For this review, use the dimensioned drawing (mm, ordinates from the lowest corner) and the shaded views. A direction names the side the tool comes from. Coordinates: 2 decimals unless noted, no trailing zeros. Loops run counter-clockwise (first coordinate to the right, second up) from the corner with the lowest first, then second, coordinate; pieces in that order, holes last. Notation, with made-up numbers: (16, 6.5) - (33, 6.5) arc R17 ccw to (33, 33.5) - close; hole circle Ø3 at (-22, 50.25). An arc over 180 degrees is marked (long way). Answer in a Markdown table with one row per item. Add a question column.
(1) We need section C-C, the plane x = 9. Write out the cut boundary in (y, z).
(2) We need section B-B, the plane x = 12.7. Write out the cut boundary in (y, z).
(3) We need section A-A, the plane y = 1.25. Write out the cut boundary in (x, z).
(4) For the marked faces 4 and 5, list the 3-axis set-ups (+Z, -Z, +X, -X, +Y, -Y) from which the entire face can be reached by the end or side of a thin tool; tool diameter is ignored.
(5) The part is to be moulded in two halves that separate along X. For the marked faces 1, 2 and 3, say which applies: released by +X, released by -X, zero draft, split by the parting line, or undercut.
(6) To check wall thickness, follow L1, parallel to X at y = 2, z = 14; L2, parallel to X at y = 5.5, z = 9.75; L3, parallel to Z at x = 13, y = 4.5. State the ranges of each line that lie inside material, in increasing order. Write a range as [from, to].
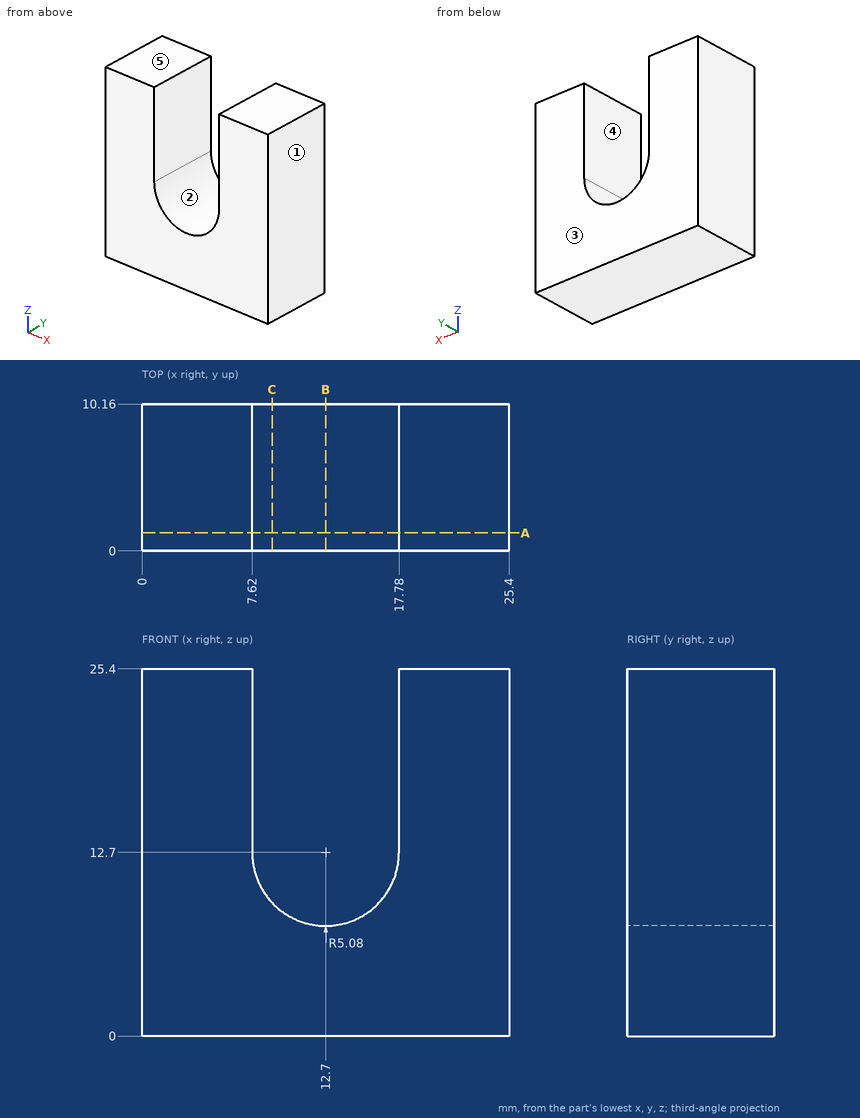
Responses:
| question | item | result |
|---|---|---|
| 1 | outline | (0, 0) - (10.16, 0) - (10.16, 9.22) - (0, 9.22) - close |
| 2 | outline | (0, 0) - (10.16, 0) - (10.16, 7.62) - (0, 7.62) - close |
| 3 | outline | (0, 0) - (25.4, 0) - (25.4, 25.4) - (17.78, 25.4) - (17.78, 12.7) arc R5.08 cw to (7.62, 12.7) - (7.62, 25.4) - (0, 25.4) - close |
| 4 | face 4 | +Z, +Y, -Y |
| 4 | face 5 | +Z, +X, -X, +Y, -Y |
| 5 | face 1 | released by +X |
| 5 | face 2 | undercut |
| 5 | face 3 | zero draft |
| 6 | L1 | x = [0, 7.62], [17.78, 25.4] |
| 6 | L2 | x = [0, 8.56], [16.84, 25.4] |
| 6 | L3 | z = [0, 7.63] |
